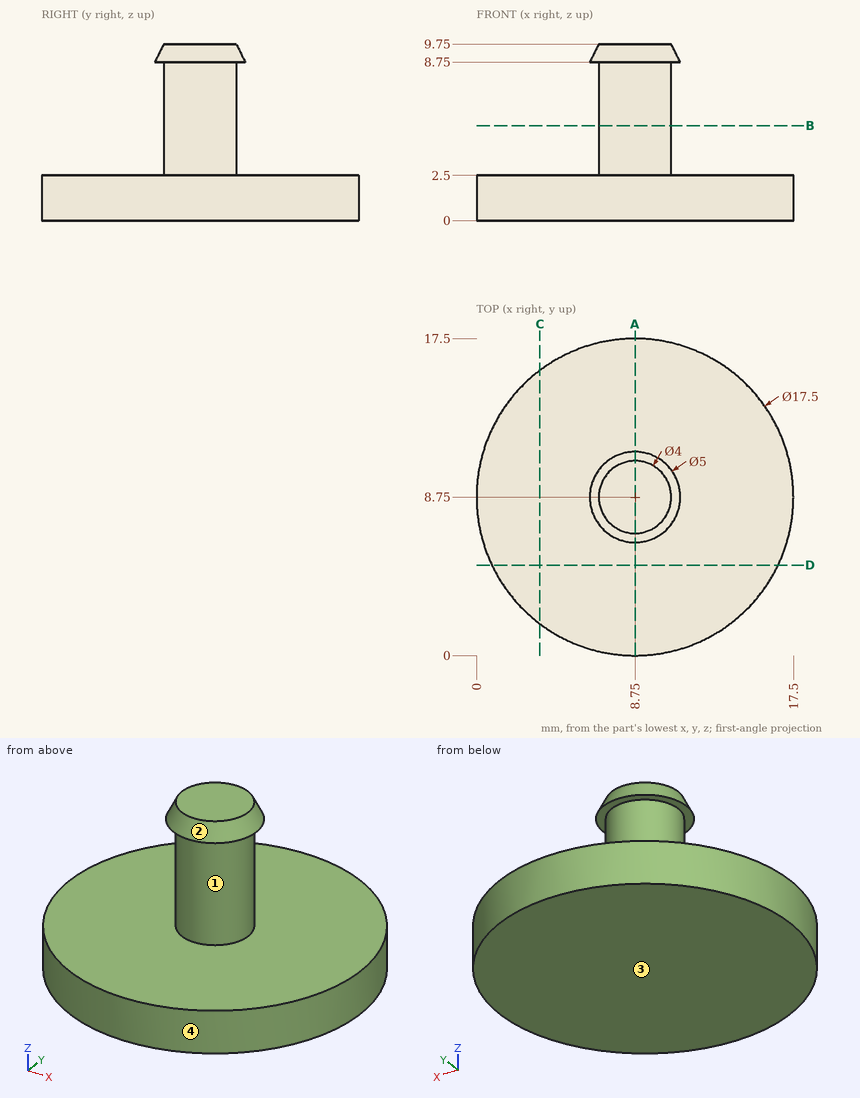
Print and shaded views of the part. All mm, measured from the part's lowest x, y and z. Round coordinates to 2 decimals unless told otherwise and drop trailing zeros. Write each loop counter-clockwise with the first axis right and the second up, starting at its lowest first coordinate (ties: lowest second). Pieces come first, ordered by that corner, then holes. Notation, with made-up numbers: M -8.5,-4 L 17.5,-4 A15 cw 17.5,9 Z; hole C 46,68.25 d10. An arc over 180 degrees is marked long. One line per question, with ' | ' between items.
(1) Probe line 1 along Z through (x, y) = (4.25, 5.75); line 2 along X through (y, z) = (1.25, 2); line 3 along Y through (x, z) = (15.75, 0.5). List the from-to ranges inside material, lowest first.
Answer key:
line 1: z = 0 to 2.5 | line 2: x = 4.24 to 13.26 | line 3: y = 3.5 to 14
(2) Two-plate mould, pull along Z, no slides. Class the marked faces 1, 2, 3 and 4: released by +Z, released by -Z, zero draft, split by the parting line, or undercut.
Answer key:
face 1: undercut | face 2: released by +Z | face 3: released by -Z | face 4: zero draft
(3) Saw through at D-D on y = 5. Write the cut outline in (x, z).
Answer key:
outline: M 0.84,0 L 16.66,0 L 16.66,2.5 L 0.84,2.5 Z
(4) Saw through at B-B on z = 5.25. Write the cut outline in (x, y), then the cut area to 3 significant figures.
Answer key:
outline: C 8.75,8.75 d4 | area: 12.6 mm^2
(5) Saw through at C-C on x = 3.5. Write the cut outline in (y, z), then the cut area to 3 significant figures.
Answer key:
outline: M 1.75,0 L 15.75,0 L 15.75,2.5 L 1.75,2.5 Z | area: 35.0 mm^2
(6) Saw through at A-A on x = 8.75. Write the cut outline in (y, z).
Answer key:
outline: M 0,0 L 17.5,0 L 17.5,2.5 L 10.75,2.5 L 10.75,8.75 L 11.25,8.75 L 10.75,9.75 L 6.75,9.75 L 6.25,8.75 L 6.75,8.75 L 6.75,2.5 L 0,2.5 Z
(7) Pin check, flat tips, straight feed: pin 1 (4 mm diameter, centred on y = 6, z = 3, fed in from +X); pin 2 (4 mm diameter, centred on x = 11, y = 4, fed in from +Z); pin 3 (2 mm diameter, centred on x = 11, z = 7, fed in from -Y). Stop position of each tip, or through.
Answer key:
pin 1: stops at x = 17.46 | pin 2: stops at z = 2.5 | pin 3: stops at y = 7.19
